```python
from build123d import *

# Parameters (mm, degrees)
F0_W     = 101.6
F0_H     = 101.6
F1_DEPTH = 3.175
F3_D     = 5.1054
F3_DEPTH = 25
F3_TIP   = 1.5338169022


# Not quite as in the source:
# - a length typed as a fraction of an inch, garbled in the dataset ("3 / 203.2 mm" for 3/8 in), is restored


with BuildPart() as f1:
    # F0 (on Right) → F1 (new body)
    with BuildSketch(Plane.YZ):
        Rectangle(F0_W, F0_H)
    extrude(amount=F1_DEPTH)

    # F3
    with Locations(Plane.YZ.offset(3.175)):
        with Locations((0, -21.9075), (-25.0825, 0), (25.0825, 0)):
            Hole(F3_D / 2, depth=F3_DEPTH)
            with Locations((0, 0, -(F3_DEPTH + F3_TIP / 2))):  # 118° drill point
                Cone(0, F3_D / 2, F3_TIP, mode=Mode.SUBTRACT)


solid = f1.part
```
Work out the finished part from the listing and answer in its coordinate system (mm). Give positions to 0.01 mm unless a question says otherwise; leave off trailing zeros. Loops run counter-clockwise (first coordinate to the right, second up) from the corner with the lowest first, then second, coordinate; pieces in that order, holes last. Notation, with made-up numbers: (-38.75, 35) -> (15.25, 35) arc R16 cw to (15.25, 49) -> close; hole circle Ø5 at (-23.5, 44.25). An arc over 180 degrees is marked (long way). Write item = value, one per line. Start each with the question number.
(1) Find the intervals of material crossed by probe 1 along Y at (x, z) = (2.5, 2); probe 2 along Y at (x, z) = (1, -0.5); probe 3 along Z at (x, y) = (2, 0), in increasing order. Write a range as from..to.
(2) Find section B-B on y = 0. Give the vertices of the cut face in (x, z) (3 decimals), and give its area (3 significant figures).
(3) Find section A-A on z = 0. Give the vertices of the cut face in (x, y) (3 decimals), and give its area (3 significant figures).
(4) The mould has two halves that part along Z. Classify faces 1 (the flat face through (2, -1, 50.8)), 2 (the flat face through (2, 50.8, -1)), 3 (the cylindrical face through (1.57, 0.55, -24.4)): +Z half, -Z half, draft (parallel to the pull), parting line (faces both ways), or undercut.
From the geometry:
q1.probe_1 = -50.8..-26.67, -23.5..23.5, 26.67..50.8
q1.probe_2 = -50.8..-27.59, -22.58..22.58, 27.59..50.8
q1.probe_3 = -50.8..-24.46, -19.35..50.8
q2.outline = (0, -50.8) -> (3.175, -50.8) -> (3.175, -24.46) -> (0, -24.46) -> close; (0, -19.355) -> (3.175, -19.355) -> (3.175, 50.8) -> (0, 50.8) -> close
q2.area = 306 mm^2
q3.outline = (0, -50.8) -> (3.175, -50.8) -> (3.175, -27.635) -> (0, -27.635) -> close; (0, -22.53) -> (3.175, -22.53) -> (3.175, 22.53) -> (0, 22.53) -> close; (0, 27.635) -> (3.175, 27.635) -> (3.175, 50.8) -> (0, 50.8) -> close
q3.area = 290 mm^2
q4.face_1 = +Z half
q4.face_2 = draft
q4.face_3 = undercut
